from build123d import *

# Parameters (mm, degrees)
F0_W     = 58.42
F0_H     = 58.42
F0_R     = 2.4765
F0_R_2   = 19.05
F1_DEPTH = 3.048
F2_R     = 5.08
F3_R     = 5.08


with BuildPart() as f1:
    # F0 (on Top) → F1 (new body)
    with BuildSketch(Plane.XY):
        Rectangle(F0_W, F0_H)
        with Locations((-23.573172, -23.573172)):
            Circle(F0_R, mode=Mode.SUBTRACT)
        Circle(F0_R_2, mode=Mode.SUBTRACT)
        with Locations((23.573172, -23.573172)):
            Circle(F0_R, mode=Mode.SUBTRACT)
        with Locations((-23.573172, 23.573172)):
            Circle(F0_R, mode=Mode.SUBTRACT)
        with Locations((23.573172, 23.573172)):
            Circle(F0_R, mode=Mode.SUBTRACT)
    extrude(amount=F1_DEPTH)

    # F2
    f2_edges = [f1.edges().sort_by_distance(p)[0] for p in [
        (-29.21, 29.21, 1.524),
    ]]
    fillet(f2_edges, radius=F2_R)

    # F3
    f3_edges = [f1.edges().sort_by_distance(p)[0] for p in [
        (29.21, 29.21, 1.524),
        (29.21, -29.21, 1.524),
        (-29.21, -29.21, 1.524),
    ]]
    fillet(f3_edges, radius=F3_R)


solid = f1.part
Verification items for the finished model (mm, model axes). Coordinates: 2 decimals unless noted, no trailing zeros. Loops run counter-clockwise (first coordinate to the right, second up) from the corner with the lowest first, then second, coordinate; pieces in that order, holes last. Notation, with made-up numbers: (-29.75, 79) -> (21.25, 79) arc R26 ccw to (21.25, 95) -> close; hole circle Ø9 at (4.25, 69). An arc over 180 degrees is marked (long way). Answer as a JSON object with one key per item and string values. Group by question number.
Item 1: Sectioned sample at C-C on z = 1.5. Record the boundary of the cut face in (x, y), plus the area to 3 significant figures.
Item 2: Sectioned sample at A-A on x = 0. Record the boundary of the cut face in (y, z), plus the area to 3 significant figures.
Item 3: Mould release check, pull along X, two halves, no side actions. Record for faces 1 (the cylindrical face through (27.682, 27.761, 1.545)), 2 (the cylindrical face through (-27.761, -27.682, 1.545)), 3 (the cylindrical face through (21.1, -23.46, 1.5)): +X half, -X half, draft (parallel to the pull), parting line (faces both ways), or undercut.
Item 4: Scan lines: probe 1 along X at (y, z) = (-23.5, 1.45); probe 2 along Y at (x, z) = (0, 2); probe 3 along Y at (x, z) = (-21.5, 0.25). Record each from-to range of solid material in increasing order.
Item 5: Depth check by flat-ended pin: pin 1 (4 mm diameter, centred on x = -23.57, y = -23.57, fed in from -Z). Enter the tip coordinate at first touch or a pass-through.
Evaluation:
{
 "1": {"outline": "(-29.21, -24.13) arc R5.08 ccw to (-24.13, -29.21) -> (24.13, -29.21) arc R5.08 ccw to (29.21, -24.13) -> (29.21, 24.13) arc R5.08 ccw to (24.13, 29.21) -> (-24.13, 29.21) arc R5.08 ccw to (-29.21, 24.13) -> close; hole circle Ø4.95 at (-23.57, -23.57); hole circle Ø4.95 at (-23.57, 23.57); hole circle Ø38.1 at (0, 0); hole circle Ø4.95 at (23.57, -23.57); hole circle Ø4.95 at (23.57, 23.57)", "area": "2,170 mm²"},
 "2": {"outline": "(-29.21, 0) -> (-19.05, 0) -> (-19.05, 3.05) -> (-29.21, 3.05) -> close; (19.05, 0) -> (29.21, 0) -> (29.21, 3.05) -> (19.05, 3.05) -> close", "area": "61.9 mm²"},
 "3": {"face 1": "+X half", "face 2": "-X half", "face 3": "undercut"},
 "4": {"probe 1": "x = -29.21 to -26.05, -21.1 to 21.1, 26.05 to 29.21", "probe 2": "y = -29.21 to -19.05, 19.05 to 29.21", "probe 3": "y = -29.21 to -24.93, -22.22 to 22.22, 24.93 to 29.21"},
 "5": {"pin 1": "passes through"}
}
